Check sheet for the modelled part. Datum: model origin and axes. Units: mm. Coordinates: 2 decimals unless noted, no trailing zeros. Loops run counter-clockwise (first coordinate to the right, second up) from the corner with the lowest first, then second, coordinate; pieces in that order, holes last.
```python
from build123d import *

# Parameters (mm, degrees)
CUT_EXTRUDE1_DEPTH = 0.5


with BuildPart() as part:
    # Sketch1 → Revolve1 (revolve)
    with BuildSketch(Plane.XY):
        with BuildLine():
            Line((0, 1.61), (1.34, 1.61))
            ThreePointArc((1.34, 1.61), (2.337020561, 1.197020561), (2.75, 0.2))
            Line((2.75, 0.2), (2.75, 0))
            Line((2.75, 0), (1.5, 0))
            Line((1.5, 0), (1.5, -10))
            Line((1.5, -10), (0, -10))
            Line((0, -10), (0, 1.61))
        make_face()
    revolve(axis=Axis((0, 9.083769969, 0), (0, -1, 0)))

    # Sketch2 → Cut-Extrude1 (cut)
    with BuildSketch(Plane(origin=(0, 1.61, 0), x_dir=(1, 0, 0), z_dir=(0, 1, 0))):
        Polygon((0.62654248, 1.085203409), (-0.62654248, 1.085203409), (-1.253084961, 0), (-0.62654248, -1.085203409), (0.62654248, -1.085203409), (1.253084961, 0), align=None)
    extrude(amount=-CUT_EXTRUDE1_DEPTH, mode=Mode.SUBTRACT)


solid = part.part
```
1) Section check A-A on y = -6.75. Enter the section's corners in (x, z), plus the area to 3 significant figures.
Answer sheet:
outline: circle Ø3 at (0, 0)
area: 7.07 mm2
2) Depth check by flat-ended pin: pin 1 (1.5 mm diameter, centred on x = 0.5, y = -6.5, fed in from -Z); pin 2 (2.5 mm diameter, centred on x = 0, z = 0.5, fed in from +Y); pin 3 (2 mm diameter, centred on y = -2.5, z = 2, fed in from +X); pin 4 (0.6 mm diameter, centred on x = -0.5, y = 1.5, fed in from -Z). Enter the tip coordinate at first touch or a pass-through.
Answer sheet:
pin 1: stops at z = -1.5
pin 2: stops at y = 1.61
pin 3: stops at x = 1.12
pin 4: stops at z = -2.29
3) Mould release check, pull along X, two halves, no side actions. Record for faces 1 (the flat face through (0, -10, 0)), 2 (the cylindrical face through (-1.5, -5.07, 0.07)), 3 (the flat face through (0, 1.11, 0)): +X half, -X half, draft (parallel to the pull), parting line (faces both ways), or undercut.
Answer sheet:
face 1: draft
face 2: parting line
face 3: undercut
4) Scan lines: line 1 (Y direction, x = 0.9, z = 0.5); line 2 (X direction, y = -1.25, z = 0.1); line 3 (Y direction, x = -1.2, z = -1.8). Record each from-to range of solid material in increasing order.
Answer sheet:
line 1: y = -10 to 1.11
line 2: x = -1.5 to 1.5
line 3: y = 0 to 1.34
